Verification items for the finished model (mm, model axes). Face numbers are marked on the shaded views. Coordinates: 2 decimals unless noted, no trailing zeros. Order: outer loops, then holes, each group sorted by start corner. A loop starts at its lowest first (then second) coordinate and runs counter-clockwise, first axis right, second up.
Q1. Cross-section at A-A, the plane y = 10. Record the boundary of the cut face in (x, z).
Q2. Draft check along X on the marked faces 1 and 2. Enter one of: pulls with the +X half, pulls with the -X half, needs draft (parallel to the pull), parting line crosses it, or undercut.
Q3. Depth check by flat-ended pin: P1, Ø1, axis at x = -12.5, z = 3, coming from the +Y side; P2, Ø1, axis at x = 8, z = 3.5, coming from the -Y side; P3, Ø1.5, axis at y = -6, z = 2.5, coming from the +X side. Enter the tip coordinate at first touch or a pass-through.
Q4. Thickness scan on line 1 (Y direction, x = 0, z = 2.75); line 2 (Y direction, x = 0, z = 4.25); line 3 (X direction, y = -22, z = 0.75). Record the ranges inside material, lowest first.
Q5. Cross-section at B-B, the plane y = -14. Count the separate pieces of the cut face and the enclosed holes in it, and give its area (3 significant figures).
Q6. Cross-section at D-D, the plane y = -1. Record the boundary of the cut face in (x, z), and give its area (3 significant figures).
from build123d import *

# Parameters (mm, degrees)
F0_R     = 11.049
F1_DEPTH = 6.35
F2_SIZE  = 2.54
F3_DEPTH = 6.35


with BuildPart() as f1:
    # F0 (on Top) → F1 (new body)
    with BuildSketch(Plane.XY):
        with BuildLine():
            ThreePointArc((0, 11.049), (-7.812823, -7.812823), (11.049, 0))
            ThreePointArc((11.049, 0), (7.812823, 7.812823), (0, 11.049))
        make_face()
        with BuildLine():
            ThreePointArc((13.97, 0), (9.878282, 9.878282), (0, 13.97))
            ThreePointArc((0, 13.97), (-9.878282, -9.878282), (13.97, 0))
        make_face()
        with BuildLine():
            ThreePointArc((0, 11.049), (7.812823, 7.812823), (11.049, 0))
            ThreePointArc((11.049, 0), (-7.812823, -7.812823), (0, 11.049))
        make_face(mode=Mode.SUBTRACT)
        with BuildLine():
            ThreePointArc((13.338323, 29.080812), (8.280673, 21.982845), (0, 19.264128))
            ThreePointArc((0, 19.264128), (-8.280673, 21.982845), (-13.338323, 29.080812))
            ThreePointArc((-13.338323, 29.080812), (-15.574662, 8.992035), (-31.853884, -2.989079))
            ThreePointArc((-31.853884, -2.989079), (-20.05689, -5.706502), (-14.811599, -16.617064))
            ThreePointArc((-14.811599, -16.617064), (-15.770499, -21.703533), (-18.51556, -26.091733))
            ThreePointArc((-18.51556, -26.091733), (0, -17.984071), (18.51556, -26.091733))
            ThreePointArc((18.51556, -26.091733), (16.683224, -9.632064), (31.853884, -2.989079))
            ThreePointArc((31.853884, -2.989079), (15.574662, 8.992035), (13.338323, 29.080812))
        make_face()
        with BuildLine():
            ThreePointArc((13.97, 0), (-9.878282, -9.878282), (0, 13.97))
            ThreePointArc((0, 13.97), (9.878282, 9.878282), (13.97, 0))
        make_face(mode=Mode.SUBTRACT)
        with BuildLine():
            ThreePointArc((11.049, 33.234128), (-7.812823, 41.046951), (0, 22.185128))
            ThreePointArc((0, 22.185128), (7.812823, 25.421305), (11.049, 33.234128))
        make_face()
        with BuildLine():
            ThreePointArc((-13.338323, 29.080812), (-8.280673, 21.982845), (0, 19.264128))
            ThreePointArc((0, 19.264128), (8.280673, 21.982845), (13.338323, 29.080812))
            ThreePointArc((13.338323, 29.080812), (13.811178, 31.133589), (13.97, 33.234128))
            ThreePointArc((13.97, 33.234128), (-2.100538, 47.045306), (-13.338323, 29.080812))
        make_face()
        with BuildLine():
            ThreePointArc((11.049, 33.234128), (7.812823, 25.421305), (0, 22.185128))
            ThreePointArc((0, 22.185128), (-7.812823, 41.046951), (11.049, 33.234128))
        make_face(mode=Mode.SUBTRACT)
        with BuildLine():
            ThreePointArc((-31.853884, -2.989079), (-15.574662, 8.992035), (-13.338323, 29.080812))
            Line((-13.338323, 29.080812), (-31.853884, -2.989079))
        make_face()
        with BuildLine():
            Line((31.853884, -2.989079), (13.338323, 29.080812))
            ThreePointArc((13.338323, 29.080812), (15.574662, 8.992035), (31.853884, -2.989079))
        make_face()
        with BuildLine():
            ThreePointArc((-14.811599, -16.617064), (-20.05689, -5.706502), (-31.853884, -2.989079))
            ThreePointArc((-31.853884, -2.989079), (-40.879974, -23.602064), (-18.51556, -26.091733))
            ThreePointArc((-18.51556, -26.091733), (-15.770499, -21.703533), (-14.811599, -16.617064))
        make_face()
        with Locations((-28.781599, -16.617064)):
            Circle(F0_R, mode=Mode.SUBTRACT)
        with BuildLine():
            ThreePointArc((42.751599, -16.617064), (39.692161, -7.892355), (31.853884, -2.989079))
            ThreePointArc((31.853884, -2.989079), (16.683224, -9.632064), (18.51556, -26.091733))
            ThreePointArc((18.51556, -26.091733), (33.868068, -29.628164), (42.751599, -16.617064))
        make_face()
        with Locations((28.781599, -16.617064)):
            Circle(F0_R, mode=Mode.SUBTRACT)
        with BuildLine():
            ThreePointArc((18.51556, -26.091733), (0, -17.984071), (-18.51556, -26.091733))
            Line((-18.51556, -26.091733), (18.51556, -26.091733))
        make_face()
    extrude(amount=F1_DEPTH)

    # F2
    f2_edges = [f1.edges().sort_by_distance(p)[0] for p in [
        (0, -26.091733, 6.35),
        (-22.596104, 13.045866, 6.35),
        (22.596104, 13.045866, 6.35),
        (-40.879974, -23.602064, 6.35),
        (40.879974, -23.602064, 6.35),
        (0, 47.204128, 6.35),
        (0, 47.204128, 0),
        (-22.596104, 13.045866, 0),
        (-40.879974, -23.602064, 0),
        (0, -26.091733, 0),
        (40.879974, -23.602064, 0),
        (22.596104, 13.045866, 0),
    ]]
    chamfer(f2_edges, length=F2_SIZE)

    # F0 (on Top) → F3 (join)
    with BuildSketch(Plane.XY):
        with BuildLine():
            ThreePointArc((13.97, 0), (9.878282, 9.878282), (0, 13.97))
            ThreePointArc((0, 13.97), (-9.878282, -9.878282), (13.97, 0))
        make_face()
        with BuildLine():
            ThreePointArc((0, 11.049), (7.812823, 7.812823), (11.049, 0))
            ThreePointArc((11.049, 0), (-7.812823, -7.812823), (0, 11.049))
        make_face(mode=Mode.SUBTRACT)
    extrude(amount=F3_DEPTH)


solid = f1.part
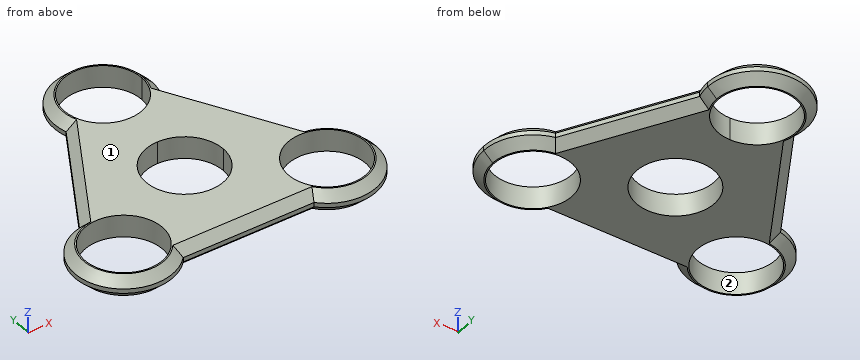
Check values:
1. outline: (-24.35, 2.54) - (-21.42, 0) - (-4.7, 0) - (-4.7, 6.35) - (-21.42, 6.35) - (-24.35, 3.81) - close; (4.7, 0) - (21.42, 0) - (24.35, 2.54) - (24.35, 3.81) - (21.42, 6.35) - (4.7, 6.35) - close
2. face 1: needs draft
2. face 2: undercut
3. P1: stops at y = 40.39
3. P2: stops at y = -26.09
3. P3: stops at x = 38.67
4. line 1: y = -26.09 to -11.05, 11.05 to 22.19, 44.28 to 47.2
4. line 2: y = -25.65 to -11.05, 11.05 to 22.19, 44.28 to 46.76
4. line 3: x = -39.71 to -38.43, -19.13 to 19.13, 38.43 to 39.71
5. separate pieces: 3
5. enclosed holes: 0
5. area: 254 mm2
6. outline: (-30.71, 2.54) - (-27.77, 0) - (-11, 0) - (-11, 6.35) - (-27.77, 6.35) - (-30.71, 3.81) - close; (11, 0) - (27.77, 0) - (30.71, 2.54) - (30.71, 3.81) - (27.77, 6.35) - (11, 6.35) - close
6. area: 235 mm2
